Geometry: final body of the model. Coordinates: model frame, mm. Face numbers are marked on the shaded views. A direction names the side the tool comes from. Coordinates: 2 decimals unless noted, no trailing zeros. Loops run counter-clockwise (first coordinate to the right, second up) from the corner with the lowest first, then second, coordinate; pieces in that order, holes last. Notation, with made-up numbers: (42, -2.5) -> (93, -2.5) arc R26 ccw to (93, 12.5) -> close; hole circle Ø11 at (-36, -35.5). An arc over 180 degrees is marked (long way). One line per item, written item: value. Start each with the question number.
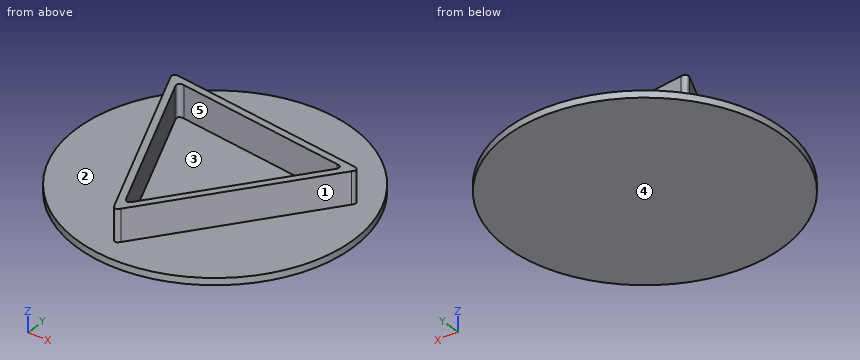
from build123d import *

# Parameters (mm, degrees)
F0_R        = 32
F1_DEPTH    = 1.6
F2_DEPTH    = 1.6
F3_DEPTH    = 9
F4_T1_DEPTH = 7.4
F4_T3_DEPTH = 11.7301270189


# Not quite as in the source:
# - a fillet or chamfer that OpenCascade refuses, or shapes differently, is made with other operations: its cross-section is extruded or revolved along the edge and cut away or added


with BuildPart() as f1:
    # F0 (on Top) → F1 (new body)
    with BuildSketch(Plane.XY):
        Circle(F0_R)
        Polygon((-3.2203362492, -27.6128490823), (-22.3032606516, 16.5953175417), (25.5235969007, 11.0175315406), align=None, mode=Mode.SUBTRACT)
        Polygon((25.5235969007, 11.0175315406), (-22.3032606516, 16.5953175417), (-3.2203362492, -27.6128490823), align=None)
        Polygon((-2.8496500622, -24.434391634), (-19.7359788499, 14.6850651628), (22.5856289122, 9.7493264712), align=None, mode=Mode.SUBTRACT)
    extrude(amount=F1_DEPTH)

    # F0 (on Top) → F2 (join)
    with BuildSketch(Plane.XY):
        Polygon((22.5856289122, 9.7493264712), (-19.7359788499, 14.6850651628), (-2.8496500622, -24.434391634), align=None)
    extrude(amount=F2_DEPTH)

    # F0 (on Top) → F3 (join)
    with BuildSketch(Plane.XY):
        Polygon((25.5235969007, 11.0175315406), (-22.3032606516, 16.5953175417), (-3.2203362492, -27.6128490823), align=None)
        Polygon((-2.8496500622, -24.434391634), (-19.7359788499, 14.6850651628), (22.5856289122, 9.7493264712), align=None, mode=Mode.SUBTRACT)
    extrude(amount=F3_DEPTH)

    # F4: fillet of radius 1 on 6 edges, made by hand

    # F4_s2 → F4_t1 (join)
    with BuildSketch(Plane.XY.offset(1.6)):
        with BuildLine():
            add(Edge.make_bspline(
                [(-3.5360861918, -22.844169813), (-2.8496500622, -24.434391634), (-1.8156956324, -23.0448095972)],
                knots=[0, 0, 0, 1, 1, 1], degree=2, weights=[1, 1, 1]))
            Line((-1.8156956324, -23.0448095972), (-2.8496500622, -24.434391634))
            Line((-2.8496500622, -24.434391634), (-3.5360861918, -22.844169813))
        make_face()
        with BuildLine():
            add(Edge.make_bspline(
                [(20.8652383527, 9.9499662554), (22.5856289122, 9.7493264712), (21.5516744823, 8.3597444344)],
                knots=[0, 0, 0, 1, 1, 1], degree=2, weights=[1, 1, 1]))
            Line((21.5516744823, 8.3597444344), (22.5856289122, 9.7493264712))
            Line((22.5856289122, 9.7493264712), (20.8652383527, 9.9499662554))
        make_face()
        with BuildLine():
            add(Edge.make_bspline(
                [(-19.0495427204, 13.0948433418), (-19.7359788499, 14.6850651628), (-18.0155882905, 14.4844253786)],
                knots=[0, 0, 0, 1, 1, 1], degree=2, weights=[1, 1, 1]))
            Line((-18.0155882905, 14.4844253786), (-19.7359788499, 14.6850651628))
            Line((-19.7359788499, 14.6850651628), (-19.0495427204, 13.0948433418))
        make_face()
    extrude(amount=F4_T1_DEPTH)

    # F4_s4 → F4_t3 (cut)
    with BuildSketch(Plane.XY.offset(1.6)):
        with BuildLine():
            add(Edge.make_bspline(
                [(-3.9067723788, -26.0226272613), (-3.2203362492, -27.6128490823), (-2.1863818193, -26.2232670455)],
                knots=[0, 0, 0, 1, 1, 1], degree=2, weights=[1, 1, 1]))
            Line((-2.1863818193, -26.2232670455), (-3.2203362492, -27.6128490823))
            Line((-3.2203362492, -27.6128490823), (-3.9067723788, -26.0226272613))
        make_face()
        with BuildLine():
            add(Edge.make_bspline(
                [(23.8032063413, 11.2181713248), (25.5235969007, 11.0175315406), (24.4896424709, 9.6279495038)],
                knots=[0, 0, 0, 1, 1, 1], degree=2, weights=[1, 1, 1]))
            Line((24.4896424709, 9.6279495038), (25.5235969007, 11.0175315406))
            Line((25.5235969007, 11.0175315406), (23.8032063413, 11.2181713248))
        make_face()
        with BuildLine():
            add(Edge.make_bspline(
                [(-20.5828700921, 16.3946777575), (-22.3032606516, 16.5953175417), (-21.616824522, 15.0050957207)],
                knots=[0, 0, 0, 1, 1, 1], degree=2, weights=[1, 1, 1]))
            Line((-21.616824522, 15.0050957207), (-22.3032606516, 16.5953175417))
            Line((-22.3032606516, 16.5953175417), (-20.5828700921, 16.3946777575))
        make_face()
    extrude(amount=F4_T3_DEPTH, mode=Mode.SUBTRACT)


solid = f1.part
1. Pin query (flat end, axial travel): pin 1 Ø1.5 at (y, z) = (-5.5, 7) entering from +X; pin 2 Ø8 at (x, y) = (-10, 23) entering from +Z; pin 3 Ø2 at (y, z) = (4, 6.5) entering from +X. Return the tip coordinate at first contact, or that it passes through.
2. Section B-B on x = 0. Return the cut outline in (y, z), plus the area to 3 significant figures.
3. Section D-D on x = -24.5. Return the cut outline in (y, z), plus the area to 3 significant figures.
4. Line query: L1, parallel to Z at x = 27.5, y = -2.5; L2, parallel to Y at x = 19, z = 6.5; L3, parallel to X at y = -2, z = 7.5. Output: solid intervals per line, ascending. Write a range as [from, to].
5. Section C-C on y = 28.5. Return the cut outline in (x, z), plus the area to 3 significant figures.
6. Section A-A on y = -5. Return the cut outline in (x, z), plus the area to 3 significant figures.
7. Set-up query: the marked faces 4 and 5. Return all of +Z, -Z, +X, -X, +Y, -Y with unobstructed straight access to the full face (end or side cutting, diameter ignored); none if empty.
8. Draft query along X for the marked faces 1, 2 and 3. Return one class per face: released by +X, released by -X, zero draft, split by the parting line, or undercut.
Checks:
1. pin 1: x = 13.79
1. pin 2: z = 1.6
1. pin 3: x = 21.05
2. outline: (-32, 0) -> (32, 0) -> (32, 1.6) -> (13.99, 1.6) -> (13.99, 9) -> (12.38, 9) -> (12.38, 1.6) -> (-20.6, 1.6) -> (-20.6, 9) -> (-23.28, 9) -> (-23.28, 1.6) -> (-32, 1.6) -> close
2. area: 134 mm²
3. outline: (-20.59, 0) -> (20.59, 0) -> (20.59, 1.6) -> (-20.59, 1.6) -> close
3. area: 65.9 mm²
4. L1: [0, 1.6]
4. L2: [2.25, 4.93], [10.17, 11.78]
4. L3: [-14.28, -12.53], [13.84, 15.84]
5. outline: (-14.55, 0) -> (14.55, 0) -> (14.55, 1.6) -> (-14.55, 1.6) -> close
5. area: 46.6 mm²
6. outline: (-31.61, 0) -> (31.61, 0) -> (31.61, 1.6) -> (13.61, 1.6) -> (13.61, 9) -> (11.61, 9) -> (11.61, 1.6) -> (-11.24, 1.6) -> (-11.24, 9) -> (-12.98, 9) -> (-12.98, 1.6) -> (-31.61, 1.6) -> close
6. area: 129 mm²
7. face 4: -Z, +X, -X, +Y, -Y
7. face 5: +Z
8. face 1: released by +X
8. face 2: zero draft
8. face 3: undercut
